Geometry check sheet. Reference: the model listing, model coordinates, mm. A direction names the side the tool comes from. Round coordinates to 2 decimals unless told otherwise and drop trailing zeros. Order: outer loops, then holes, each group sorted by start corner. A loop starts at its lowest first (then second) coordinate and runs counter-clockwise, first axis right, second up.
(1) Thickness scan on L1, parallel to Z at x = 40, y = 21.5; L2, parallel to Y at x = 7, z = -30; L3, parallel to X at y = 70.5, z = -115.5. Record the ranges inside material, lowest first.
(2) Cross-section at A-A on x = -7.5. Enter the section's corners in (y, z), and give its area (3 significant figures).
(3) Draft check along Z on faces 1 (the face through (34.32, 19.545, 2.535)), 2 (the face through (26, 40, -122)), 3 (the face through (12.613, 68.586, -57.611)). Enter one of: pulls with the +Z half, pulls with the -Z half, needs draft (parallel to the pull), parting line crosses it, or undercut.
(4) Cross-section at B-B on z = -26. Enter the section's corners in (x, y), and give its area (3 significant figures).
(5) Gauge pin test, flat ends, axial feed: P1, Ø1.4, axis at x = 13.21, y = 14.75, coming from the +Z side; P2, Ø2.5, axis at x = 39.81, y = 15.12, coming from the -Z side. Record the tip position at first contact, or that the pin passes through.
(6) Cross-section at C-C on y = 35. Enter the section's corners in (x, z).
(7) Set-up check for faces 4 (the face through (12.73, 18.81, 2.46)), 5 (the face through (20.244, 56.796, -3.628)), 6 (the face through (18.828, 59.273, -3.776)): record each of +Z, -Z, +X, -X, +Y, -Y from which the full face is reachable in a straight line by a thin tool's end or side.
from build123d import *

# Parameters (mm, degrees)
AUFSATZ_LINEAR_AUSTRAGEN1_DEPTH = 5
AUFSATZ_LINEAR_AUSTRAGEN2_DEPTH = 5
AUFSATZ_LINEAR_AUSTRAGEN3_DEPTH = 127
VERRUNDUNG1_R                   = 5
SKIZZE4_R                       = 1.15
SCHNITT_LINEAR_AUSTRAGEN1_DEPTH = 160.018146459
VERRUNDUNG2_R                   = 5
SKIZZE5_W                       = 10.358999457
SKIZZE5_H                       = 18.2
AUFSATZ_LINEAR_AUSTRAGEN4_DEPTH = 3
SKIZZE6_R                       = 3.5
SCHNITT_LINEAR_AUSTRAGEN2_DEPTH = 146.462570096
VERRUNDUNG4_R                   = 3


with BuildPart() as part:
    # Skizze1 → Aufsatz-Linear austragen1 (new body)
    with BuildSketch(Plane.XY):
        Polygon((-19.239846421, 13.575566883), (6.456161255, 83.889632397), (50.130587288, 7.506440349), align=None)
        Polygon((-11.237544669, 20.906014898), (7.458044946, 72.064269891), (39.234154141, 16.490313423), align=None, mode=Mode.SUBTRACT)
    extrude(amount=AUFSATZ_LINEAR_AUSTRAGEN1_DEPTH)



with BuildPart() as body_2:
    # Skizze2 → Aufsatz-Linear austragen2 (new body)
    with BuildSketch(Plane(origin=(0, 0, -117), x_dir=(-1, 0, 0), z_dir=(0, 0, -1))):
        Polygon((-50.130587288, 7.506440349), (19.239846421, 13.575566883), (-6.456161255, 83.889632397), align=None)
        Polygon((-39.234154141, 16.490313423), (11.237544669, 20.906014898), (-7.458044946, 72.064269891), align=None, mode=Mode.SUBTRACT)
    extrude(amount=AUFSATZ_LINEAR_AUSTRAGEN2_DEPTH)


with BuildPart() as part_1:
    add(part.part)

    add(body_2.part)  # Aufsatz-Linear austragen3 merges body 2
    # Skizze3 → Aufsatz-Linear austragen3 (add, through all)
    with BuildSketch(Plane.XY.offset(5)):
        Polygon((6.456161255, 83.889632397), (-0.408718311, 65.10470683), (16.38354695, 66.527402895), align=None)
    extrude(amount=-AUFSATZ_LINEAR_AUSTRAGEN3_DEPTH)

    # Verrundung1
    verrundung1_edges = [part_1.edges().sort_by_distance(p)[0] for p in [
        (-11.237544669, 20.906014898, 2.5),
        (39.234154141, 16.490313423, 2.5),
        (50.130587288, 7.506440349, -119.5),
        (-19.239846421, 13.575566883, -119.5),
        (39.234154141, 16.490313423, -119.5),
        (-11.237544669, 20.906014898, -119.5),
        (-19.239846421, 13.575566883, 2.5),
        (50.130587288, 7.506440349, 2.5),
    ]]
    fillet(verrundung1_edges, radius=VERRUNDUNG1_R)

    # Skizze4 → Schnitt-Linear austragen1 (cut, through all)
    with BuildSketch(Plane.XY.offset(5)):
        with Locations((-12.521530051, 18.969329152)):
            Circle(SKIZZE4_R)
        with Locations(Location((39.809827396, 15.116890366, 0), (0, 0, 180))):
            Circle(SKIZZE4_R)
        with Locations(Location((13.212061367, 14.751672192, 0), (0, 0, 180))):
            Circle(SKIZZE4_R)
    extrude(amount=-SCHNITT_LINEAR_AUSTRAGEN1_DEPTH, mode=Mode.SUBTRACT)

    # Verrundung2
    # the kernel refuses this fillet: 5 mm, written as the material it takes off along each edge
    with BuildSketch(Plane(origin=(6.456161255, 83.889632397, 31.907592949), x_dir=(-0.34324397830304476, -0.9392462783310345, 0), z_dir=(0, 0, -1))) as verrundung2_piece_1:
        with BuildLine():
            CenterArc((VERRUNDUNG2_R * 2.15260743589, -VERRUNDUNG2_R), VERRUNDUNG2_R, 90, 130.165278403)
            Line((VERRUNDUNG2_R * 1.38842039617, -VERRUNDUNG2_R * 1.64499470411), (0, 0))
            Line((0, 0), (VERRUNDUNG2_R * 2.15260743589, 0))
        make_face()
    extrude(amount=180.815185897, mode=Mode.SUBTRACT)
    with BuildSketch(Plane(origin=(-0.408718311, 65.10470683, 19.589879441), x_dir=(0.34324397830304404, 0.9392462783310347, 0), z_dir=(0, 0, -1))) as verrundung2_piece_2_section:
        with BuildLine():
            CenterArc((VERRUNDUNG2_R * 1.56719035525, VERRUNDUNG2_R), VERRUNDUNG2_R, 155.082639201, 114.917360799)
            Line((VERRUNDUNG2_R * 0.660273957752, VERRUNDUNG2_R * 1.42131063118), (0, 0))
            Line((0, 0), (VERRUNDUNG2_R * 1.56719035525, 0))
        make_face()
    verrundung2_piece_2 = extrude(amount=156.179758881, mode=Mode.PRIVATE)
    verrundung2_piece_2 = split(verrundung2_piece_2, bisect_by=Plane(origin=(5.223636013, 65.950075885, 2.5), z_dir=(0.9392462783310345, -0.34324397830304465, 0)), keep=Keep.TOP, mode=Mode.PRIVATE)
    add(verrundung2_piece_2, mode=Mode.SUBTRACT)
    with BuildSketch(Plane(origin=(-0.408718311, 65.10470683, 0), x_dir=(0.34324397830304504, 0.9392462783310342, 0), z_dir=(0, 0, -1)), Plane(origin=(16.38354695, 66.527402895, 0), x_dir=(-0.9964301882569208, -0.08442085009212626, 0), z_dir=(0, 0, -1))) as verrundung2_piece_3:
        with BuildLine():
            CenterArc((VERRUNDUNG2_R * 1.56719035525, VERRUNDUNG2_R), VERRUNDUNG2_R, 155.082639201, 114.917360799)
            Line((VERRUNDUNG2_R * 0.660273957752, VERRUNDUNG2_R * 1.42131063118), (0, 0))
            Line((0, 0), (VERRUNDUNG2_R * 1.56719035525, 0))
        make_face()
    extrude(amount=117, mode=Mode.SUBTRACT)
    with BuildSketch(Plane(origin=(16.38354695, 66.527402895, 19.589879441), x_dir=(-0.9964301882569208, -0.08442085009212626, 0), z_dir=(0, 0, -1))) as verrundung2_piece_4_section:
        with BuildLine():
            CenterArc((VERRUNDUNG2_R * 1.56719035525, VERRUNDUNG2_R), VERRUNDUNG2_R, 155.082639201, 114.917360799)
            Line((VERRUNDUNG2_R * 0.660273957752, VERRUNDUNG2_R * 1.42131063118), (0, 0))
            Line((0, 0), (VERRUNDUNG2_R * 1.56719035525, 0))
        make_face()
    verrundung2_piece_4 = extrude(amount=156.179758881, mode=Mode.PRIVATE)
    verrundung2_piece_4 = split(verrundung2_piece_4, bisect_by=Plane(origin=(10.689250835, 66.413140789, 2.5), z_dir=(-0.868111475056711, -0.4963692847818663, 0)), keep=Keep.TOP, mode=Mode.PRIVATE)
    add(verrundung2_piece_4, mode=Mode.SUBTRACT)

    # Skizze5 → Aufsatz-Linear austragen4 (add)
    with BuildSketch(Plane(origin=(41.013843737, 23.450919458, 0), x_dir=(0, 0, -1), z_dir=(0.868111475056711, 0.4963692847818664, 0))):
        with Locations((5.179499729, 48.356864154)):
            Rectangle(SKIZZE5_W, SKIZZE5_H)
    extrude(amount=-AUFSATZ_LINEAR_AUSTRAGEN4_DEPTH)

    # Skizze6 → Schnitt-Linear austragen2 (cut, through all)
    with BuildSketch(Plane(origin=(41.013843737, 23.450919458, 0), x_dir=(0, 0, -1), z_dir=(0.868111475056711, 0.4963692847818664, 0))):
        with Locations(Location((3.929999457, 45.606864154, 0), (0, 0, 90))):
            Circle(SKIZZE6_R)
    extrude(amount=-SCHNITT_LINEAR_AUSTRAGEN2_DEPTH, mode=Mode.SUBTRACT)

    # Verrundung4
    verrundung4_edges = [part_1.edges().sort_by_distance(p)[0] for p in [
        (20.225774942, 56.785699777, -10.358999457),
    ]]
    fillet(verrundung4_edges, radius=VERRUNDUNG4_R)


solid = part_1.part
Found:
1. L1: z = -122 to -117, 0 to 5
1. L2: y = 65.75 to 77.04
1. L3: x = 1.98 to 13.14
2. outline: (12.55, -122) - (21.48, -122) - (21.48, -117) - (12.55, -117) - close; (12.55, 0) - (21.48, 0) - (21.48, 5) - (12.55, 5) - close; (31.13, -122) - (45.7, -122) - (45.7, -117) - (31.13, -117) - close; (31.13, 0) - (45.7, 0) - (45.7, 5) - (31.13, 5) - close
2. area: 235 mm2
3. face 1: needs draft
3. face 2: pulls with the -Z half
3. face 3: undercut
4. outline: (2.28, 72.46) arc R5 ccw to (7.4, 65.77) - (8.58, 65.87) arc R5 ccw to (12.49, 73.33) - (11.8, 74.55) arc R5 ccw to (2.76, 73.78) - close
4. area: 99.2 mm2
5. P1: passes through
5. P2: stops at z = -122
6. outline: (-11.41, -122) - (-6.09, -122) - (-6.09, -117) - (-11.41, -117) - close; (-11.41, 0) - (-6.09, 0) - (-6.09, 5) - (-11.41, 5) - close; (28.65, -122) - (34.41, -122) - (34.41, -117) - (28.65, -117) - close; (28.65, 0) - (34.41, 0) - (34.41, 5) - (28.65, 5) - close
7. face 4: +Z, -Z
7. face 5: +X, -Y
7. face 6: none
